The listing builds one solid part. Answer for the finished solid, in the listing's coordinates (mm). Face numbers are marked on the shaded views. Coordinates: 2 decimals unless noted, no trailing zeros. Write each loop counter-clockwise with the first axis right and the second up, starting at its lowest first coordinate (ties: lowest second). Pieces come first, ordered by that corner, then holes. Notation, with made-up numbers: M -40,60.25 L -16,60.25 A18 cw -16,95.25 Z; hole C 0.5,86 d1. An arc over 180 degrees is marked long. Answer as a JSON object with one key per item and string values. Group by question number.
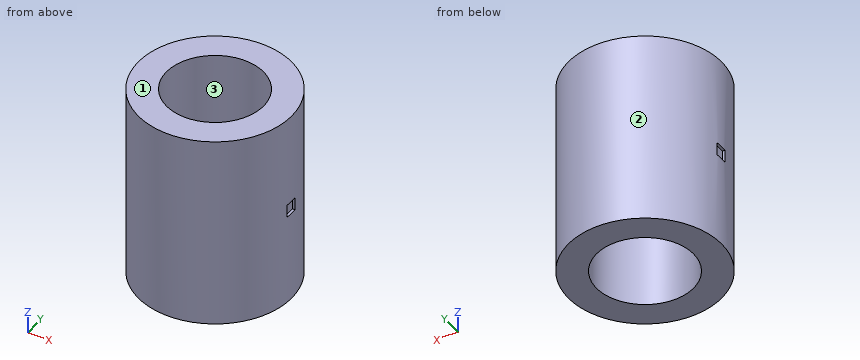
from build123d import *

# Parameters (mm, degrees)
CROQUIS1_R              = 3
CROQUIS1_R_2            = 1.9
SALIENTE_EXTRUIR1_DEPTH = 7.6
CROQUIS3_W              = 0.5
CROQUIS3_H              = 0.5
CORTAR_EXTRUIR1_DEPTH   = 0.1


with BuildPart() as part:
    # Croquis1 → Saliente-Extruir1 (new body)
    with BuildSketch(Plane.XY):
        with Locations(Location((0, 0, 0), (0, 0, 180))):
            Circle(CROQUIS1_R)
        with Locations(Location((0, 0, 0), (0, 0, 180))):
            Circle(CROQUIS1_R_2, mode=Mode.SUBTRACT)
    extrude(amount=SALIENTE_EXTRUIR1_DEPTH)

    # Croquis3 → Cortar-Extruir1 (cut)
    with BuildSketch(Plane.ZY.offset(3)):
        with Locations((3.8, 0)):
            Rectangle(CROQUIS3_W, CROQUIS3_H)
    cortar_extruir1 = extrude(amount=-CORTAR_EXTRUIR1_DEPTH, mode=Mode.SUBTRACT)

    # Simetría1: Cortar-Extruir1 across plane
    add(cortar_extruir1.mirror(Plane(origin=(0, 0, 0), x_dir=(0, 0, 1), z_dir=(1, 0, 0))), mode=Mode.SUBTRACT)


solid = part.part
Item 1: A cutting plane is placed at B-B, the plane x = 0. Write down the section's boundary in (y, z).
Item 2: A cutting plane is placed at A-A, the plane y = 0. Write down the section's boundary in (x, z).
Item 3: A cutting plane is placed at C-C, the plane z = 3.25. Write down the section's boundary in (x, y).
Item 4: For a pull along Y with two mould halves and no side action, classify the marked faces 1, 2 and 3 as +Y half, -Y half, draft (parallel to the pull), parting line (faces both ways), or undercut.
Item 5: A cutting plane is placed at D-D, the plane y = 0.7. Write down the section's boundary in (x, z).
Item 6: Consider L1, parallel to Y at x = 0, z = 4.25; L2, parallel to X at y = 1.1, z = 0.5; L3, parallel to X at y = -1.7, z = 6. Determine where each line is inside the solid, lowest interval first. Write a range as from..to.
Item 7: A flat-ended cylindrical pin translates along its axis: pin 1 Ø0.6 at (y, z) = (0, 4) entering from -X. Find the tip coordinate at first contact, or state that the pin passes through.
Answer:
{
 "1": {"outline": "M -3,0 L -1.9,0 L -1.9,7.6 L -3,7.6 Z; M 1.9,0 L 3,0 L 3,7.6 L 1.9,7.6 Z"},
 "2": {"outline": "M -3,0 L -1.9,0 L -1.9,7.6 L -3,7.6 L -3,4.05 L -2.9,4.05 L -2.9,3.55 L -3,3.55 Z; M 1.9,0 L 3,0 L 3,3.55 L 2.9,3.55 L 2.9,4.05 L 3,4.05 L 3,7.6 L 1.9,7.6 Z"},
 "3": {"outline": "C 0,0 d6; hole C 0,0 d3.8"},
 "4": {"face 1": "draft", "face 2": "parting line", "face 3": "undercut"},
 "5": {"outline": "M -2.92,0 L -1.77,0 L -1.77,7.6 L -2.92,7.6 Z; M 1.77,0 L 2.92,0 L 2.92,7.6 L 1.77,7.6 Z"},
 "6": {"L1": "-3..-1.9, 1.9..3", "L2": "-2.79..-1.55, 1.55..2.79", "L3": "-2.47..-0.85, 0.85..2.47"},
 "7": {"pin 1": "x = -3"}
}
